Can you work these out from the model? Positions are in its coordinate system, mm. A direction names the side the tool comes from. Coordinates: 2 decimals unless noted, no trailing zeros. Order: outer loops, then holes, each group sorted by start corner. A loop starts at its lowest first (then second) coordinate and runs counter-clockwise, first axis right, second up. Notation, with made-up numbers: (78.25, -14) -> (116.25, -14) arc R16 ccw to (116.25, 4) -> close; hole circle Ø2 at (70.25, 81). An arc over 180 degrees is marked (long way). Answer in a Markdown table with one row per item.
```python
from build123d import *

# Parameters (mm, degrees)
F0_W      = 52.8
F0_H      = 52.8
F0_W_2    = 42.8
F0_H_2    = 42.8
F1_DEPTH  = 39.4
F2_W      = 52.8
F2_H      = 52.8
F3_DEPTH  = 10
F4_W      = 10
F4_H      = 10
F5_DEPTH  = 25
F6_W      = 10
F6_H      = 10
F7_DEPTH  = 10
F9_D      = 5.5
F9_DEPTH  = 9
F9_TIP    = 1.6523667023
F11_D     = 5.5
F11_DEPTH = 9
F11_TIP   = 1.6523667023


with BuildPart() as f1:
    # F0 (on Top) → F1 (new body)
    with BuildSketch(Plane.XY):
        with Locations((30.4056062862, 18.5175239619)):
            Rectangle(F0_W, F0_H)
        with Locations((30.4056062862, 18.5175239619)):
            Rectangle(F0_W_2, F0_H_2, mode=Mode.SUBTRACT)
    extrude(amount=F1_DEPTH)

    # F2 (on Top) → F3 (join)
    with BuildSketch(Plane.XY):
        with Locations((30.3273436148, 18.6009341)):
            Rectangle(F2_W, F2_H)
    extrude(amount=-F3_DEPTH)

    # F4 (on face) → F5 (cut)
    with BuildSketch(Plane.YZ.offset(56.8056062862)):
        with Locations((18.5175239619, 5)):
            Rectangle(F4_W, F4_H)
    extrude(amount=-F5_DEPTH, mode=Mode.SUBTRACT)

    # F6 (on face) → F7 (join)
    with BuildSketch(Plane.XY.offset(39.4)):
        with Locations((30.4056062862, 49.9175239619)):
            Rectangle(F6_W, F6_H)
    extrude(amount=-F7_DEPTH)

    # F9
    with Locations(Plane.XY.offset(39.4)):
        with Locations((30.4083697991, 50.0837391585)):
            Hole(F9_D / 2, depth=F9_DEPTH)
            with Locations((0, 0, -(F9_DEPTH + F9_TIP / 2))):  # 118° drill point
                Cone(0, F9_D / 2, F9_TIP, mode=Mode.SUBTRACT)

    # F11
    with Locations(Plane(origin=(0, 0, -10), x_dir=(1, 0, 0), z_dir=(0, 0, -1))):
        with Locations((30.3273436148, -19.0009341)):
            Hole(F11_D / 2, depth=F11_DEPTH)
            with Locations((0, 0, -(F11_DEPTH + F11_TIP / 2))):  # 118° drill point
                Cone(0, F11_D / 2, F11_TIP, mode=Mode.SUBTRACT)


solid = f1.part
```
(1) Will these pins go through, and if not, where does the flat tip stop? pin 1 Ø1.5 at (x, z) = (53, 5.5) entering from +Y; pin 2 Ø4 at (x, y) = (35, 9.5) entering from +Z; pin 3 Ø4 at (y, z) = (6.5, 6.5) entering from -X.
Response values:
| item | result |
|---|---|
| pin 1 | y = 44.92 |
| pin 2 | z = 0 |
| pin 3 | x = 4.01 |
(2) On a 3-axis mill with a long thin cutter (end or side, diameter ignored), from which of +Z, -Z, +X, -X, +Y, -Y can I reach the whole of each face in a straight line? I mean faces 4 (the flat face through (30, -2.882, 19)), 5 (the flat face through (3.927, 18, -5)), 6 (the flat face through (30, -7.799, -5)), 7 (the flat face through (35.406, 50, 34)), 8 (the flat face through (54, 18, 10)). Say none if no direction works.
Response values:
| item | result |
|---|---|
| face 4 | +Z |
| face 5 | +Z, -Z, -X, +Y, -Y |
| face 6 | -Z, +X, -X, -Y |
| face 7 | +Z, -Z, +X, +Y |
| face 8 | +X |
(3) Suppose I cut it at B-B (x = 53). Please give me the cut outline in (y, z).
Response values:
| item | result |
|---|---|
| outline | (-7.88, 0) -> (-7.8, 0) -> (-7.8, -10) -> (45, -10) -> (45, 0) -> (44.92, 0) -> (44.92, 39.4) -> (-7.88, 39.4) -> close; hole (13.52, 0) -> (23.52, 0) -> (23.52, 10) -> (13.52, 10) -> close |
(4) Suppose I cut it at C-C (y = 1). Please give me the cut outline in (x, z).
Response values:
| item | result |
|---|---|
| outline | (3.93, -10) -> (56.73, -10) -> (56.73, 0) -> (56.81, 0) -> (56.81, 39.4) -> (51.81, 39.4) -> (51.81, 0) -> (9.01, 0) -> (9.01, 39.4) -> (4.01, 39.4) -> (4.01, 0) -> (3.93, 0) -> close |
(5) We'd pull the mould along X, two halves only. Please class faces 1 (the flat face through (7, 17, 39.4)), 2 (the cylindrical face through (32.35, 17.14, -5.44)), 3 (the flat face through (56.806, 18, 19)): +X half, -X half, draft (parallel to the pull), parting line (faces both ways), or undercut.
Response values:
| item | result |
|---|---|
| face 1 | draft |
| face 2 | undercut |
| face 3 | +X half |
(6) Suppose I cut it at D-D (x = 46). Please give me the cut outline in (y, z), and give its area (3 significant figures).
Response values:
| item | result |
|---|---|
| outline | (-7.88, 0) -> (-7.8, 0) -> (-7.8, -10) -> (45, -10) -> (45, 0) -> (44.92, 0) -> (44.92, 39.4) -> (39.92, 39.4) -> (39.92, 0) -> (-2.88, 0) -> (-2.88, 39.4) -> (-7.88, 39.4) -> close |
| area | 922 mm2 |
(7) Suppose I cut it at A-A (z = 16). Please give me the cut outline in (x, y).
Response values:
| item | result |
|---|---|
| outline | (4.01, -7.88) -> (56.81, -7.88) -> (56.81, 44.92) -> (4.01, 44.92) -> close; hole (9.01, -2.88) -> (51.81, -2.88) -> (51.81, 39.92) -> (9.01, 39.92) -> close |
(8) I need wall thicknesses on line 1 (Y direction, x = 25.5, z = 26); line 2 (X direction, y = 5.5, z = 18); line 3 (Y direction, x = 19, z = -5.5). Which ranges of each line are inside material? Lowest first, please. Write a range as [from, to].
Response values:
| item | result |
|---|---|
| line 1 | [-7.88, -2.88], [39.92, 44.92] |
| line 2 | [4.01, 9.01], [51.81, 56.81] |
| line 3 | [-7.8, 45] |
